Design review of the part shown in the three views and the two pictorial views. Dimensions are in mm from the part's minimum x, y and z. A direction names the side the tool comes from. Coordinates: 2 decimals unless noted, no trailing zeros. Loops run counter-clockwise (first coordinate to the right, second up) from the corner with the lowest first, then second, coordinate; pieces in that order, holes last. Notation, with made-up numbers: (-25.5, 13.25) -> (-19.5, 13.25) arc R15 ccw to (-19.5, 19.25) -> close; hole circle Ø9 at (27, -3). An arc over 180 degrees is marked (long way). Use a Markdown table: item, result. Add a question column.
Q1. Draft analysis for pull direction Z (two halves, no side actions). For the marked faces 1, 2, 3 and 4, state which applies: pulls with the +Z half, pulls with the -Z half, needs draft (parallel to the pull), parting line crosses it, or undercut.
Q2. For probe 1 along X at (y, z) = (8.25, 15); probe 2 along Z at (x, y) = (19, 8); probe 3 along X at (y, z) = (3.75, 16), list the stretches that pass through material, from the lowest coordinate up.
Q3. Take a section at C-C on z = 26. Write out the cut boundary in (x, y), plus the area to 3 significant figures.
Q4. Take a section at B-B on y = 4. Write out the cut boundary in (x, z).
Q5. For the marked faces 5 and 6, list the 3-axis set-ups (+Z, -Z, +X, -X, +Y, -Y) from which the entire face can be reached by the end or side of a thin tool; tool diameter is ignored.
Q6. Clearance check with flat-ended pins moving along their axes: pin 1 Ø1.6 at (y, z) = (11.5, 15.5) entering from -X; pin 2 Ø6.5 at (x, z) = (24, 17) entering from +Y; pin 3 Ø2 at (x, z) = (14, 13) entering from +Y; pin 4 Ø1.6 at (x, z) = (37, 15) entering from +Y. State where each tip first meets the part, or that it passes through.
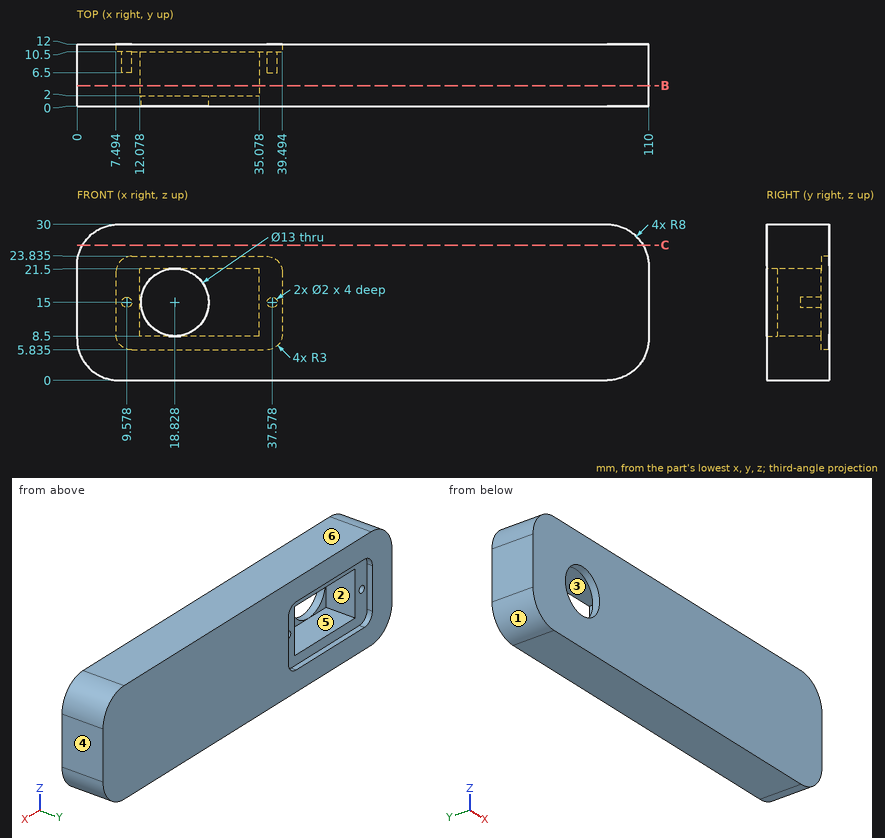
Answer list:
| question | item | result |
|---|---|---|
| 1 | face 1 | pulls with the -Z half |
| 1 | face 2 | undercut |
| 1 | face 3 | undercut |
| 1 | face 4 | needs draft |
| 2 | probe 1 | 0 to 8.58, 10.58 to 12.08, 35.08 to 36.58, 38.58 to 110 |
| 2 | probe 2 | 0 to 8.5, 21.5 to 30 |
| 2 | probe 3 | 0 to 12.08, 35.08 to 110 |
| 3 | outline | (1.07, 0) -> (108.93, 0) -> (108.93, 12) -> (1.07, 12) -> close |
| 3 | area | 1,290 mm² |
| 4 | outline | (0, 8) arc R8 ccw to (8, 0) -> (102, 0) arc R8 ccw to (110, 8) -> (110, 22) arc R8 ccw to (102, 30) -> (8, 30) arc R8 ccw to (0, 22) -> close; hole (12.08, 8.5) -> (35.08, 8.5) -> (35.08, 21.5) -> (12.08, 21.5) -> close |
| 5 | face 5 | +Y |
| 5 | face 6 | +Z, +X, -X, +Y, -Y |
| 6 | pin 1 | x = 0 |
| 6 | pin 2 | y = 2 |
| 6 | pin 3 | through |
| 6 | pin 4 | y = 10.5 |
